Source: CAD feature listing. Evaluate the final solid. Frame: model axes, mm. Face numbers are marked on the shaded views. A direction names the side the tool comes from. Round coordinates to 2 decimals unless told otherwise and drop trailing zeros. Loops run counter-clockwise (first coordinate to the right, second up) from the corner with the lowest first, then second, coordinate; pieces in that order, holes last. Notation, with made-up numbers: M 25,18 L 33,18 A11 ccw 33,37 Z; hole C 66,87 d1. An arc over 180 degrees is marked long. Answer as a JSON object with one key per item and string values.
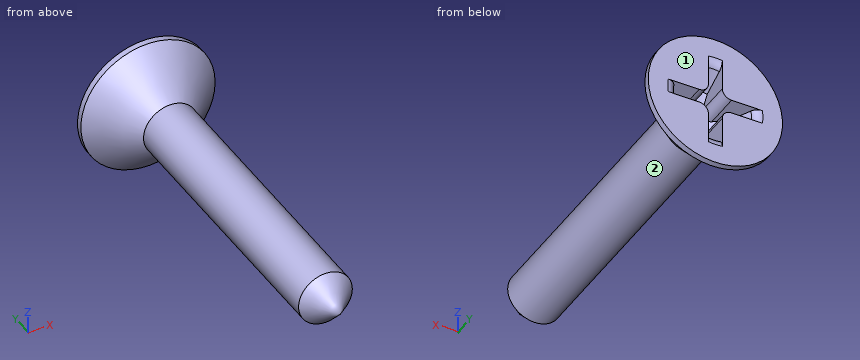
Autodesk Inventor part; units mm, degrees
ref_plane "YZ Plane" through (0, 0, 0) normal (1, 0, 0) x (0, 1, 0)
ref_plane "XZ Plane" through (0, 0, 0) normal (0, 1, 0) x (-1, 0, 0)
ref_plane "XY Plane" through (0, 0, 0) normal (0, 0, 1) x (1, 0, 0)
sketch "Sketch1" plane through (0, 0, 0) normal (0, 0, 1) x (1, 0, 0)
  line L0 (0, -2.5) -> (0, -19)
  line L1 (0, -19) -> (1.4515, -17.5485)
  line L2 (1.4515, -17.5485) -> (1.4515, -2.5)
  line L3 (1.4515, -2.5) -> (3.625, -0.3265)
  line L4 (3.625, -0.3265) -> (3.625, 0)
  line L5 (3.625, 0) -> (2.25, 0)
  line L6 (0.7598, -2.0613) -> (0, -2.5)
  line L7 (0.7598, -2.0613) -> (1.5664, -1.466)
  line L8 (1.5664, -1.466) -> (2.25, 0)
  point P0 (0, 0)
  dimension "d0" = 3.625
  dimension "d1" = 2.25
  dimension "d2" = 19
  dimension "d3" = 60
  dimension "d4" = 45
  dimension "d5" = 2.5
  dimension "d6" = 2.5
  dimension "d7" = 25
revolve "Revolution1" add sketch "Sketch1" angle 360 about axis through (0, -2.5, 0) along (0, -1, 0)
sketch "Sketch2" plane through (0, 0, 0) normal (0, 1, 0) x (1, 0, 0)
  circle A0 centre (0, 0) radius 2.25
  line L0 (0, 2.25) -> (0.375, 2.25)
  line L1 (0.375, 2.25) -> (-0.375, 2.25)
  line L2 (-0.375, 2.25) -> (-0.375, 0.875)
  line L3 (-0.875, 0.375) -> (-2.25, 0.375)
  line L4 (-2.25, 0.375) -> (-2.25, -0.375)
  line L5 (-2.25, -0.375) -> (-0.875, -0.375)
  line L6 (-0.375, -0.875) -> (-0.375, -2.25)
  line L7 (-0.375, -2.25) -> (0.375, -2.25)
  line L8 (0.375, -2.25) -> (0.375, -0.875)
  line L9 (0.875, -0.375) -> (2.25, -0.375)
  line L10 (2.25, -0.375) -> (2.25, 0.375)
  line L11 (2.25, 0.375) -> (0.875, 0.375)
  line L12 (0.375, 2.25) -> (0.375, 0.875)
  arc A1 (0.375, 0.875) -> (0.875, 0.375) centre (0.875, 0.875) ccw
  arc A2 (0.875, -0.375) -> (0.375, -0.875) centre (0.875, -0.875) ccw
  arc A3 (-0.375, -0.875) -> (-0.875, -0.375) centre (-0.875, -0.875) ccw
  arc A4 (-0.875, 0.375) -> (-0.375, 0.875) centre (-0.875, 0.875) ccw
  point P0 (0, 0)
  point P1 (-0.375, 0.375)
  point P2 (-0.375, -0.375)
  point P3 (0.375, -0.375)
  point P4 (0.375, 0.375)
  point P5 (-2.2185, -0.375)
  point P6 (-0.375, -2.2185)
  point P7 (0.375, -2.2185)
  point P8 (2.2185, -0.375)
  point P9 (2.2185, 0.375)
  point P10 (0.375, 2.2185)
  point P11 (-0.375, 2.2185)
  point P12 (-2.2185, 0.375)
  dimension "d9" = 0.375
  dimension "d10" = 0.75
  dimension "d11" = 1.875
  dimension "d12" = 1.875
  dimension "d13" = 0.75
  dimension "d14" = 1.875
  dimension "d15" = 1.875
  dimension "d16" = 0.5
extrude "Extrusion1" add sketch "Sketch2" against normal up to next contours L11 A1 L12 A0 | A0 L8 A2 L9 | L2 A4 L3 A0 | A0 L5 A3 L6
fillet "Fillet1" radius 0.5 4 edges at (-2.25, 0, 0) (0, 0, 2.25) (2.25, 0, 0) (0, 0, -2.25)
properties part number "screw EE" material "Iron, Malleable"
Item 1: Line query: probe 1 along Y at (x, z) = (1.25, -2.5); probe 2 along Z at (x, y) = (-0.5, -14). Output: solid intervals per line, ascending. Write a range as from..to.
Answer sheet:
{"probe 1": "y = -1.16..0", "probe 2": "z = -1.36..1.36"}
Item 2: Section A-A on y = -9.5. Return the cut outline in (x, z), then the cut area to 3 significant figures.
Answer sheet:
{"outline": "C 0,0 d2.9", "area": "6.62 mm²"}
Item 3: Contact query for flat-ended pins moving along their axis: pin 1 Ø1.8 at (y, z) = (-1.5, -1.5) entering from +X; pin 2 Ø0.8 at (y, z) = (-0.5, 1.5) entering from +X; pin 3 Ø0.5 at (x, y) = (1.5, -0.5) entering from -Z. Output: stop coordinate, or through.
Answer sheet:
{"pin 1": "stops at x = 3.07", "pin 2": "stops at x = 3.44", "pin 3": "stops at z = -3.38"}
Item 4: Access query for the marked faces 1 and 2. Directions: +Z, -Z, +X, -X, +Y, -Y. A direction counts if a zero-diameter tool reaches every point of the face in a straight line with its end or side. Return the directions, or none.
Answer sheet:
{"face 1": "+Z, -Z, +X, -X, +Y", "face 2": "-Y"}
